from build123d import *

# Parameters (mm, degrees)
SKETCH_1_W      = 36.8
SKETCH_1_H      = 16.7
EXTRUDE_1_DEPTH = 4.1
SKETCH_2_W      = 2.5
SKETCH_2_H      = 16.7
EXTRUDE_2_DEPTH = 3
SKETCH_3_R      = 0.2
EXTRUDE_3_DEPTH = 6.65


with BuildPart() as part:
    # 草图1 → 凸台-拉伸1 (new body)
    with BuildSketch(Plane.XY):
        with Locations((18.4, 8.35)):
            Rectangle(SKETCH_1_W, SKETCH_1_H)
    extrude(amount=EXTRUDE_1_DEPTH)

    # 草图2 → 凸台-拉伸2 (add)
    with BuildSketch(Plane.XY.offset(4.1)):
        with Locations((1.25, 8.35)):
            Rectangle(SKETCH_2_W, SKETCH_2_H)
    extrude(amount=EXTRUDE_2_DEPTH)

    # 草图3 → 凸台-拉伸3 (add)
    with BuildSketch(Plane.ZY):
        with Locations(Location((5.671300253, 15.164518481, 0), (0, 0, 180))):
            Circle(SKETCH_3_R)
        with Locations(Location((5.671300253, 12.664518481, 0), (0, 0, 180))):
            Circle(SKETCH_3_R)
        with Locations(Location((5.671300253, 10.164518481, 0), (0, 0, 180))):
            Circle(SKETCH_3_R)
        with Locations(Location((5.671300253, 7.664518481, 0), (0, 0, 180))):
            Circle(SKETCH_3_R)
        with Locations(Location((5.671300253, 5.164518481, 0), (0, 0, 180))):
            Circle(SKETCH_3_R)
        with Locations(Location((5.671300253, 2.664518481, 0), (0, 0, 180))):
            Circle(SKETCH_3_R)
    extrude(amount=EXTRUDE_3_DEPTH)


solid = part.part
Verification items for the finished model (mm, model axes). A direction names the side the tool comes from. Coordinates: 2 decimals unless noted, no trailing zeros. Loops run counter-clockwise (first coordinate to the right, second up) from the corner with the lowest first, then second, coordinate; pieces in that order, holes last. Notation, with made-up numbers: (63, 17) -> (73, 17) arc R26 ccw to (73, 36) -> close; hole circle Ø3 at (71, -8.5). An arc over 180 degrees is marked (long way). Answer as CSV lines item,"result".
1) Depth check by flat-ended pin: pin 1 (1 mm diameter, centred on x = -1.5, z = 1.5, fed in from -Y); pin 2 (1.5 mm diameter, centred on x = 4, y = 14, fed in from +Z); pin 3 (3.5 mm diameter, centred on y = 10.5, z = 6, fed in from +X). Enter the tip coordinate at first touch or a pass-through.
Found:
pin 1,"passes through"
pin 2,"stops at z = 4.1"
pin 3,"stops at x = 2.5"
2) Thickness scan on L1, parallel to X at y = 12.75, z = 1.5; L2, parallel to Z at x = 33.5, y = 4.25; L3, parallel to X at y = 9.25, z = 6.5. Record the ranges inside material, lowest first. Write a range as from..to.
Found:
L1,"x = 0..36.8"
L2,"z = 0..4.1"
L3,"x = 0..2.5"
3) Tool access check on faces 1 (the flat face through (19, 8, 4.1)), 2 (the flat face through (36.8, 8, 2)). Record the directions out of +Z, -Z, +X, -X, +Y, -Y that give a thin tool (end or side, any length) a straight path to the whole face; none if there is none.
Found:
face 1,"+Z, +X, +Y, -Y"
face 2,"+Z, -Z, +X, +Y, -Y"
4) Cross-section at A-A, the plane y = 4.5. Record the cut outline in (x, z).
Found:
outline,"(0, 0) -> (36.8, 0) -> (36.8, 4.1) -> (2.5, 4.1) -> (2.5, 7.1) -> (0, 7.1) -> close"
5) Cross-section at C-C, the plane z = 3.5. Record the cut outline in (x, y).
Found:
outline,"(0, 0) -> (36.8, 0) -> (36.8, 16.7) -> (0, 16.7) -> close"
6) Cross-section at D-D, the plane x = 13. Record the cut outline in (y, z).
Found:
outline,"(0, 0) -> (16.7, 0) -> (16.7, 4.1) -> (0, 4.1) -> close"
7) Cross-section at B-B, the plane x = -2. Record the cut outline in (y, z).
Found:
outline,"circle Ø0.4 at (2.66, 5.67); circle Ø0.4 at (5.16, 5.67); circle Ø0.4 at (7.66, 5.67); circle Ø0.4 at (10.16, 5.67); circle Ø0.4 at (12.66, 5.67); circle Ø0.4 at (15.16, 5.67)"
